Read the model definition and answer for the solid it produces. Units are mm, in the model's axes. A direction names the side the tool comes from. Coordinates: 2 decimals unless noted, no trailing zeros. Write each loop counter-clockwise with the first axis right and the second up, starting at its lowest first coordinate (ties: lowest second). Pieces come first, ordered by that corner, then holes. Notation, with made-up numbers: (15.5, 40.25) -> (56.5, 40.25) arc R15 cw to (56.5, 45.25) -> close; hole circle Ø3 at (28, -30). An arc over 180 degrees is marked (long way). Answer as a JSON object with one key per item and string values. Group by question number.
(1) Find section A-A (x = 0). Give the vertices of the cut face in (y, z), then the cut area to 3 significant figures.
(2) Which of the six approach directions +Z, -Z, +X, -X, +Y, -Y give full straight-line access (tool end or side, diameter ignored) to faces 5 (the face through (0, -31.577, 13)), 6 (the face through (0, 31.923, 13)), 7 (the face through (15, 14, 25.4))?
(3) For a pull along X with two mould halves and no side action, classify faces 1 (the face through (15.12, -11.59, -26.11)), 2 (the face through (-31.75, 0, 13)), 3 (the face through (31.75, 0, 13)), 4 (the face through (13, 15, -76.2)) as +X half, -X half, draft (parallel to the pull), parting line (faces both ways), or undercut.
(4) Flat-ended cylindrical pins translate along their axes: P1, Ø1, axis at x = 48, y = 10, coming from the +Z side; P2, Ø12.5, axis at y = 4, z = 11.5, coming from the +X side; P3, Ø7.5, axis at y = 14, z = 15, coming from the -X side; P4, Ø23, axis at x = 0, y = 0, coming from the -Z side. Find the tip coordinate at first contact, or state that the pin passes through.
(5) Find section D-D (z = -54). Give the vertices of the cut face in (x, y), then the cut area to 3 significant figures.
(6) Straight lines are drawn through the part: L1, parallel to Y at x = 0, z = -21; L2, parallel to Z at x = 39, y = 30; L3, parallel to X at y = 14.5, z = -50.5. For each, find the intervals that lie inside material, in ascending order.
(7) Find section B-B (y = 0). Give the vertices of the cut face in (x, z), then the cut area to 3 significant figures.
(8) Find section C-C (y = 25.5). Give the vertices of the cut face in (x, z), then the cut area to 3 significant figures.
from build123d import *

# Parameters (mm, degrees)
F3_W      = 63.5
F3_H      = 25.4
F4_DEPTH  = 31.75
F4_FACE_W = 63.5
F4_FACE_H = 25.4
F5_DEPTH  = 31.75
F2_R      = 63.5
F6_DEPTH  = 76.2
F7_D      = 38.1


with BuildPart() as f4:
    # F3 (on Right) → F4 (new body)
    with BuildSketch(Plane.YZ):
        with Locations((0.173381, 12.7)):
            Rectangle(F3_W, F3_H)
    extrude(amount=F4_DEPTH)

    # F4_face (on face) → F5 (join)
    with BuildSketch(Plane(origin=(0, 0.173381, 12.7), x_dir=(0, 1, 0), z_dir=(-1, 0, 0))):
        Rectangle(F4_FACE_W, F4_FACE_H)
    extrude(amount=F5_DEPTH)

    # F2 (on Top) → F6 (join)
    with BuildSketch(Plane.XY):
        Circle(F2_R)
    extrude(amount=-F6_DEPTH)

    # F7 (through all)
    with Locations(Plane.XY.offset(25.4)):
        with Locations((0, 0)):
            Hole(F7_D / 2)


solid = f4.part
Results below:
{
 "1": {"outline": "(-63.5, -76.2) -> (-19.05, -76.2) -> (-19.05, 25.4) -> (-31.58, 25.4) -> (-31.58, 0) -> (-63.5, 0) -> close; (19.05, -76.2) -> (63.5, -76.2) -> (63.5, 0) -> (31.92, 0) -> (31.92, 25.4) -> (19.05, 25.4) -> close", "area": "7,420 mm2"},
 "2": {"face 5": "+Z, +X, -X, -Y", "face 6": "+Z, +X, -X, +Y", "face 7": "+Z, +X, -X, +Y, -Y"},
 "3": {"face 1": "undercut", "face 2": "-X half", "face 3": "+X half", "face 4": "draft"},
 "4": {"P1": "stops at z = 0", "P2": "stops at x = 31.75", "P3": "stops at x = -31.75", "P4": "passes through"},
 "5": {"outline": "circle Ø127 at (0, 0); hole circle Ø38.1 at (0, 0)", "area": "11,500 mm2"},
 "6": {"L1": "y = -63.5 to -19.05, 19.05 to 63.5", "L2": "z = -76.2 to 0", "L3": "x = -61.82 to -12.36, 12.36 to 61.82"},
 "7": {"outline": "(-63.5, -76.2) -> (-19.05, -76.2) -> (-19.05, 25.4) -> (-31.75, 25.4) -> (-31.75, 0) -> (-63.5, 0) -> close; (19.05, -76.2) -> (63.5, -76.2) -> (63.5, 0) -> (31.75, 0) -> (31.75, 25.4) -> (19.05, 25.4) -> close", "area": "7,420 mm2"},
 "8": {"outline": "(-58.15, -76.2) -> (58.15, -76.2) -> (58.15, 0) -> (31.75, 0) -> (31.75, 25.4) -> (-31.75, 25.4) -> (-31.75, 0) -> (-58.15, 0) -> close", "area": "10,500 mm2"}
}
